from build123d import *

# Parameters (mm, degrees)
ESQUISSE1_W             = 67
ESQUISSE1_H             = 28
BOSS_EXTRU_1_DEPTH      = 8
ESQUISSE2_W             = 11.5
ESQUISSE2_H             = 6
ESQUISSE2_W_2           = 9
BOSS_EXTRU_2_DEPTH      = 120
ESQUISSE4_R             = 2
ENL_V_MAT_EXTRU_2_DEPTH = 3
BOSS_EXTRU_3_DEPTH      = 11.5
ESQUISSE7_W             = 5.5
ESQUISSE7_H             = 19
ENL_V_MAT_EXTRU_3_DEPTH = 120
BOSS_EXTRU_4_DEPTH      = 9
ESQUISSE9_W             = 4
ESQUISSE9_H             = 19
ENL_V_MAT_EXTRU_4_DEPTH = 120
CONG_2_R                = 2


with BuildPart() as part:
    # Esquisse1 → Boss.-Extru.1 (new body)
    with BuildSketch(Plane.XY):
        with Locations((33.5, 14)):
            Rectangle(ESQUISSE1_W, ESQUISSE1_H)
    extrude(amount=BOSS_EXTRU_1_DEPTH)

    # Esquisse2 → Boss.-Extru.2 (add)
    with BuildSketch(Plane.XY.offset(8)):
        with Locations((5.75, 22)):
            Rectangle(ESQUISSE2_W, ESQUISSE2_H)
        with Locations((62.5, 22)):
            Rectangle(ESQUISSE2_W_2, ESQUISSE2_H)
    extrude(amount=BOSS_EXTRU_2_DEPTH)

    # Esquisse4 → Enlèv. mat.-Extru.2 (cut)
    with BuildSketch(Plane.XY.offset(8)):
        with Locations((6.83, 14)):
            Circle(ESQUISSE4_R)
        with Locations(Location((61.17, 14, 0), (0, 0, 180))):
            Circle(ESQUISSE4_R)
    extrude(amount=-ENL_V_MAT_EXTRU_2_DEPTH, mode=Mode.SUBTRACT)

    # Esquisse5 → Boss.-Extru.3 (add)
    with BuildSketch(Plane.ZY):
        Polygon((8, 0), (68, 19), (52.210526316, 19), (8, 5), align=None)
    extrude(amount=-BOSS_EXTRU_3_DEPTH)

    # Esquisse7 → Enlèv. mat.-Extru.3 (cut)
    with BuildSketch(Plane.XY.offset(128)):
        with Locations((5.75, 9.5)):
            Rectangle(ESQUISSE7_W, ESQUISSE7_H)
    extrude(amount=-ENL_V_MAT_EXTRU_3_DEPTH, mode=Mode.SUBTRACT)

    # Esquisse8 → Boss.-Extru.4 (add)
    with BuildSketch(Plane(origin=(67, 0, 0), x_dir=(0, 0, -1), z_dir=(1, 0, 0))):
        Polygon((-8, 0), (-8, 5), (-52.210526316, 19), (-68, 19), align=None)
    extrude(amount=-BOSS_EXTRU_4_DEPTH)

    # Esquisse9 → Enlèv. mat.-Extru.4 (cut)
    with BuildSketch(Plane.XY.offset(128)):
        with Locations((62.5, 9.5)):
            Rectangle(ESQUISSE9_W, ESQUISSE9_H)
    extrude(amount=-ENL_V_MAT_EXTRU_4_DEPTH, mode=Mode.SUBTRACT)

    # Congé2
    cong_2_edges = [part.edges().sort_by_distance(p)[0] for p in [
        (67, 19, 30.105263158),
        (58, 19, 30.105263158),
        (58, 25, 68),
        (58, 19, 98),
        (67, 19, 98),
        (67, 25, 68),
        (58, 22, 128),
        (62.5, 19, 128),
        (67, 22, 128),
        (62.5, 25, 128),
        (0, 19, 98),
        (11.5, 19, 98),
        (11.5, 25, 68),
        (0, 25, 68),
        (5.75, 19, 128),
        (11.5, 22, 128),
        (5.75, 25, 128),
        (0, 22, 128),
        (11.5, 19, 30.105263158),
        (0, 19, 30.105263158),
    ]]
    fillet(cong_2_edges, radius=CONG_2_R)


solid = part.part
Geometry check sheet. Reference: the model listing, model coordinates, mm. A direction names the side the tool comes from. Give positions to 0.01 mm unless a question says otherwise; leave off trailing zeros. Loops run counter-clockwise (first coordinate to the right, second up) from the corner with the lowest first, then second, coordinate; pieces in that order, holes last. Notation, with made-up numbers: (49.5, -5) -> (99.5, -5) arc R12 cw to (99.5, 5) -> close; hole circle Ø5 at (-30, -15). An arc over 180 degrees is marked (long way). Answer in a Markdown table with one row per item. Add a question column.
1) Material ranges on probe 1 along X at (y, z) = (14, 7.3); probe 2 along Y at (x, z) = (6.83, 6.15); probe 3 along X at (y, z) = (21.25, 110.5), recorded low to high. Write a range as from..to.
2) Draft check along X on faces 1 (the face through (67, 14, 40)), 2 (the face through (33, 14, 8)), 3 (the face through (33, 28, 4)). Enter one of: pulls with the +X half, pulls with the -X half, needs draft (parallel to the pull), parting line crosses it, or undercut.
3) Cross-section at A-A on y = 6.5. Record the boundary of the cut face in (x, z).
4) Cross-section at B-B on z = 112.5. Record the boundary of the cut face in (x, y).
5) Set-up check for faces 4 (the face through (6, 25, 66)), 5 (the face through (8.5, 11, 34)), 6 (the face through (11.5, 16, 49)), 7 (the face through (5.4, 15.4, 6.5)): record each of +Z, -Z, +X, -X, +Y, -Y from which the full face is reachable in a straight line by a thin tool's end or side.
6) Gauge pin test, flat ends, axial feed: P1, Ø5.5, axis at x = 62, z = 40, coming from the +Y side; P2, Ø8, axis at x = 6, z = 93, coming from the -Y side; P3, Ø8.5, axis at x = 30, y = 17.5, coming from the +Z side. Record the tip position at first contact, or that the pin passes through.
7) Cross-section at D-D on z = 28. State how many separate pieces and enclosed holes the cut face has, and give its area (3 significant figures).
8) Cross-section at C-C on x = 6.83. Record the boundary of the cut face in (y, z), and give its area (3 significant figures).
Outcome:
| question | item | result |
|---|---|---|
| 1 | probe 1 | x = 0..4.83, 8.83..59.17, 63.17..67 |
| 1 | probe 2 | y = 0..12, 16..28 |
| 1 | probe 3 | x = 0..11.5, 58..67 |
| 2 | face 1 | pulls with the +X half |
| 2 | face 2 | undercut |
| 2 | face 3 | needs draft |
| 3 | outline | (0, 0) -> (67, 0) -> (67, 8) -> (0, 8) -> close; (0, 12.74) -> (3, 12.74) -> (3, 28.53) -> (0, 28.53) -> close; (8.5, 12.74) -> (11.5, 12.74) -> (11.5, 28.53) -> (8.5, 28.53) -> close; (58, 12.74) -> (60.5, 12.74) -> (60.5, 28.53) -> (58, 28.53) -> close; (64.5, 12.74) -> (67, 12.74) -> (67, 28.53) -> (64.5, 28.53) -> close |
| 4 | outline | (0, 21) arc R2 ccw to (2, 19) -> (9.5, 19) arc R2 ccw to (11.5, 21) -> (11.5, 23) arc R2 ccw to (9.5, 25) -> (2, 25) arc R2 ccw to (0, 23) -> close; (58, 21) arc R2 ccw to (60, 19) -> (65, 19) arc R2 ccw to (67, 21) -> (67, 23) arc R2 ccw to (65, 25) -> (60, 25) arc R2 ccw to (58, 23) -> close |
| 5 | face 4 | +Z, +X, -X, +Y |
| 5 | face 5 | +Z, -Y |
| 5 | face 6 | +Z, +Y, -Y |
| 5 | face 7 | none |
| 6 | P1 | stops at y = 25 |
| 6 | P2 | stops at y = 19 |
| 6 | P3 | stops at z = 8 |
| 7 | separate pieces | 6 |
| 7 | enclosed holes | 0 |
| 7 | area | 171 mm^2 |
| 8 | outline | (0, 0) -> (28, 0) -> (28, 8) -> (25, 8) -> (25, 126) arc R2 ccw to (23, 128) -> (21, 128) arc R2 ccw to (19, 126) -> (19, 8) -> (16, 8) -> (16, 5) -> (12, 5) -> (12, 8) -> (0, 8) -> close |
| 8 | area | 930 mm^2 |
